Verification items for the finished model (mm, model axes). Give positions to 0.01 mm unless a question says otherwise; leave off trailing zeros. Order: outer loops, then holes, each group sorted by start corner. A loop starts at its lowest first (then second) coordinate and runs counter-clockwise, first axis right, second up. Notation, with made-up numbers: (57, 1.25) - (70, 1.25) arc R22 ccw to (70, 16.25) - close; hole circle Ø4 at (75, -28). An arc over 180 degrees is marked (long way). Answer as a JSON object with one key per item and string values.
Autodesk Inventor part; units mm, degrees
ref_plane "YZ Plane" through (0, 0, 0) normal (1, 0, 0) x (0, 1, 0)
ref_plane "XZ Plane" through (0, 0, 0) normal (0, 1, 0) x (-1, 0, 0)
ref_plane "XY Plane" through (0, 0, 0) normal (0, 0, 1) x (1, 0, 0)
sketch "Skizze1" plane through (0, 0, 0) normal (0, 0, 1) x (1, 0, 0)
  line L0 (-3.85, 4.425) -> (3.85, 4.425)
  line L1 (3.85, 4.425) -> (3.85, -4.425)
  line L2 (3.85, -4.425) -> (-3.85, -4.425)
  line L3 (-3.85, -4.425) -> (-3.85, 4.425)
  line L4 (-3.85, 4.425) -> (3.85, -4.425) construction
  point P0 (0, 0)
  point P1 (0, 0)
  dimension "d0" = 7.7
  dimension "d1" = 8.85
extrude "Extrusion2" add sketch "Skizze1" along normal blind 1.11
sketch "Skizze2" plane through (0, 0, 1.11) normal (0, 0, 1) x (1, 0, 0)
  line L0 (3.85, 4.425) -> (-3.85, 4.425) construction
  line L1 (-3.85, 4.425) -> (-3.85, 3.125) construction
  line L2 (-3.85, 4.425) -> (-3.85, -4.425) construction
  line L3 (-3.85, 3.125) -> (3.85, 3.125) construction
  line L4 (3.85, -4.425) -> (3.85, 4.425) construction
  line L5 (-3.85, 3.125) -> (-3.05, 3.125) construction
  line L6 (3.85, 3.125) -> (3.05, 3.125) construction
  line L7 (-3.05, 3.125) -> (-2.6, 3.125) construction
  circle A0 centre (-2.6, 3.125) radius 0.45
  circle A1 centre (-0.05, 3.125) radius 0.45
  circle A2 centre (2.5, 3.125) radius 0.45
  circle A3 centre (5.05, 3.125) radius 0.45
  circle A4 centre (7.6, 3.125) radius 0.45
  circle A5 centre (10.15, 3.125) radius 0.45
  line L8 (-3.85, -4.425) -> (-3.85, -3.125) construction
  line L9 (-3.85, -3.125) -> (3.85, -3.125) construction
  line L10 (-3.85, -3.125) -> (-2.6, -3.125) construction
  circle A6 centre (-2.6, -3.125) radius 0.45
  circle A7 centre (-0.05, -3.125) radius 0.45
  line L11 (-1.3, -3.125) -> (6.4, -3.125) construction
  circle A8 centre (2.5, -3.125) radius 0.45
  line L12 (1.25, -3.125) -> (8.95, -3.125) construction
  circle A9 centre (5.05, -3.125) radius 0.45
  line L13 (3.8, -3.125) -> (11.5, -3.125) construction
  circle A10 centre (7.6, -3.125) radius 0.45
  line L14 (6.35, -3.125) -> (14.05, -3.125) construction
  circle A11 centre (10.15, -3.125) radius 0.45
  line L15 (8.9, -3.125) -> (16.6, -3.125) construction
  line L16 (3.05, 3.125) -> (2.6, 3.125)
  point P0 (0, 0)
  dimension "d6" = 1.3
  dimension "d7" = 0.8
  dimension "d8" = 0.8
  dimension "d9" = 0.45
  dimension "d10" = 0.9
  dimension "d13" = 2.55
  dimension "d20" = 1.3
  dimension "d21" = 1.25
  dimension "d22" = 0.9
  dimension "d25" = 2.55
  dimension "d30" = 0.45
extrude "Extrusion3" cut sketch "Skizze2" against normal blind 1.11 contours A0 | A1 | A2 | A3 | A4 | A5 | A6 | A7 | A8 | A10 | A11
sketch "Skizze3" plane through (0, 0, 1.11) normal (0, 0, 1) x (1, 0, 0)
  line L0 (3.8509, -4.4242) -> (-3.85, -4.425) construction
  line L1 (-3.85, -4.425) -> (-3.8509, 4.4242) construction
  line L2 (-3.8509, 4.4242) -> (3.85, 4.425) construction
  line L3 (3.85, 4.425) -> (3.8509, -4.4242) construction
  point P0 (0, 0)
  point P1 (3.85, 4.425)
  point P2 (-3.85, -4.425)
decal "Aufkleber1"
properties part number "chip_gross"
(1) Release check for a two-part mould opening along Y. For faces 1 (the cylindrical face through (-0.11, 3.57, 0.56)), 2 (the flat face through (0, 0, 1.11)), 3 (the flat face through (0.1, -4.425, 0.5)), 4 (the flat face through (-0.1, 4.425, 0.5)) record: pulls with the +Y half, pulls with the -Y half, needs draft (parallel to the pull), parting line crosses it, or undercut.
Computed values:
{"face 1": "undercut", "face 2": "needs draft", "face 3": "pulls with the -Y half", "face 4": "pulls with the +Y half"}
(2) Section check D-D (x = 0). Record the cut outline in (y, z) (3 decimals), then the cut area to 3 significant figures.
Computed values:
{"outline": "(-4.425, 0) - (-3.572, 0) - (-3.572, 1.11) - (-4.425, 1.11) - close; (-2.678, 0) - (2.678, 0) - (2.678, 1.11) - (-2.678, 1.11) - close; (3.572, 0) - (4.425, 0) - (4.425, 1.11) - (3.572, 1.11) - close", "area": "7.84 mm²"}
(3) Section check C-C (y = 3.25). Record the cut outline in (x, z).
Computed values:
{"outline": "(-3.85, 0) - (-3.03, 0) - (-3.03, 1.11) - (-3.85, 1.11) - close; (-2.17, 0) - (-0.48, 0) - (-0.48, 1.11) - (-2.17, 1.11) - close; (0.38, 0) - (2.07, 0) - (2.07, 1.11) - (0.38, 1.11) - close; (2.93, 0) - (3.85, 0) - (3.85, 1.11) - (2.93, 1.11) - close"}
(4) Section check A-A (x = 2.5). Record the cut outline in (y, z) (3 decimals), then the cut area to 3 significant figures.
Computed values:
{"outline": "(-4.425, 0) - (-3.575, 0) - (-3.575, 1.11) - (-4.425, 1.11) - close; (-2.675, 0) - (2.675, 0) - (2.675, 1.11) - (-2.675, 1.11) - close; (3.575, 0) - (4.425, 0) - (4.425, 1.11) - (3.575, 1.11) - close", "area": "7.83 mm²"}
(5) Material ranges on line 1 along Y through (x, z) = (2.5, 0.9) (3 decimals); line 2 along X through (y, z) = (-3.5, 0.5), recorded low to high. Write a range as [from, to].
Computed values:
{"line 1": "y = [-4.425, -3.575], [-2.675, 2.675], [3.575, 4.425]", "line 2": "x = [-3.85, -2.85], [-2.35, -0.3], [0.2, 2.25], [2.75, 3.85]"}
(6) Section check B-B (z = 0.55). Record the cut outline in (x, y) (3 decimals), then the cut area to 3 significant figures.
Computed values:
{"outline": "(-3.85, -4.425) - (3.85, -4.425) - (3.85, 4.425) - (-3.85, 4.425) - close; hole circle Ø0.9 at (-2.6, -3.125); hole circle Ø0.9 at (-2.6, 3.125); hole circle Ø0.9 at (-0.05, -3.125); hole circle Ø0.9 at (-0.05, 3.125); hole circle Ø0.9 at (2.5, -3.125); hole circle Ø0.9 at (2.5, 3.125)", "area": "64.3 mm²"}
